The model under review builds one solid part; all positions refer to its coordinate system, in mm. Face numbers are marked on the shaded views. A direction names the side the tool comes from. Coordinates: 2 decimals unless noted, no trailing zeros. Write each loop counter-clockwise with the first axis right and the second up, starting at its lowest first coordinate (ties: lowest second). Pieces come first, ordered by that corner, then holes.
1) For line 1 (X direction, y = -3, z = 0); line 2 (Z direction, x = 0, y = -3.75); line 3 (Y direction, x = 0, z = 0.95), list the stretches that pass through material, from the lowest coordinate up.
2) For P1, Ø6, axis at y = -6.5, z = -4, coming from the +X side; P2, Ø1.5, axis at x = -1, z = 3.5, coming from the +Y side; P3, Ø6, axis at x = 4, z = -4, coming from the -Y side, all flat-tipped, find the tip position at first contact; note any pin that passes through.
3) Add section D-D, the plane x = 0. Give the number of separate pieces and of enclosed holes in the cut face, then the cut area to 4 significant figures.
4) Add section A-A, the plane y = -5.25. State the section outline as (x, z) points, then the cut area to 3 significant figures.
5) Add section C-C, the plane z = 2.25. State the section outline as (x, y) points.
6) Add section B-B, the plane x = 1.5. State the section outline as (y, z) points, then the cut area to 3 significant figures.
7) Machinability: for the marked faces 4, 5, 6 and 7, which of the approach directions +Z, -Z, +X, -X, +Y, -Y give a long, thin tool a straight path to every point of the face, cutting with its end or side? Answer none if there is none.
8) Mouldability with a two-part tool opening along Z and no side actions: class the marked faces 1, 2 and 3 as released by +Z, released by -Z, zero draft, split by the parting line, or undercut.
Autodesk Inventor part; units mm, degrees
ref_plane "YZ Plane" through (0, 0, 0) normal (1, 0, 0) x (0, 1, 0)
ref_plane "XZ Plane" through (0, 0, 0) normal (0, 1, 0) x (-1, 0, 0)
ref_plane "XY Plane" through (0, 0, 0) normal (0, 0, 1) x (1, 0, 0)
sketch "Sketch1" plane through (0, 0, 0) normal (0, 1, 0) x (-1, 0, 0)
  circle A0 centre (0, 0) radius 5.25
  dimension "d0" = 10.5
extrude "Extrusion1" add sketch "Sketch1" against normal blind 12
sketch "Sketch2" plane through (0, 0, 0) normal (0, 1, 0) x (1, 0, 0)
  circle A0 centre (0, 0) radius 4
  dimension "d3" = 8
extrude "Extrusion2" cut sketch "Sketch2" against normal blind 10
sketch "Sketch3" plane through (0, 0, 0) normal (0, 0, 1) x (1, 0, 0)
  point P0 (0, 0)
sketch "Sketch4" plane through (0, 0, 0) normal (0, 0, 1) x (1, 0, 0)
  circle A0 centre (0, 0) radius 0.75
  circle A1 centre (0, 0) radius 1.25
  line L0 (-1.25, 0) -> (-1.25, -10)
  line L1 (-1.25, -10) -> (1.25, -10)
  line L2 (1.25, -10) -> (1.25, 0)
  dimension "d6" = 1.5
  dimension "d7" = 2.5
  dimension "d8" = 10
extrude "Extrusion3" add sketch "Sketch4" along normal mid plane 2 contours L2 L1 L0 A1
sketch "Sketch5" plane through (0, 0, 1) normal (0, 0, 1) x (1, 0, 0)
  circle A0 centre (0, 0) radius 0.75
  circle A1 centre (0, 0) radius 1.25
extrude "Extrusion4" add sketch "Sketch5" along normal mid plane 0.5
extrude "Extrusion5" add sketch "Sketch5" along normal blind 0.5
mirror "Mirror1" about plane through (0, 0, 0) normal (0, 0, 1) of "Extrusion4"
sketch "Sketch6" plane through (0, -12, 0) normal (0, -1, 0) x (1, 0, 0)
  circle A0 centre (0, 0) radius 5.25
extrude "Extrusion6" cut sketch "Sketch6" against normal blind 4
sketch "Sketch7" plane through (0, -8, 0) normal (0, -1, 0) x (1, 0, 0)
  circle A0 centre (0, 0) radius 4
extrude "Extrusion7" add sketch "Sketch7" against normal blind 1
sketch "Sketch8" plane through (0, -8, 0) normal (0, -1, 0) x (1, 0, 0)
  circle A0 centre (0, 0) radius 1.25
  dimension "d19" = 2.5
extrude "Extrusion8" add sketch "Sketch8" along normal blind 2
sketch "Sketch9" plane through (0, 0, 0) normal (0, 0, 1) x (1, 0, 0)
  line L0 (-1.25, -10) -> (1.25, -10)
  line L1 (1.25, -8) -> (-1.25, -8)
  circle A0 centre (0, -9) radius 0.6
  point P0 (0, 0)
  point P1 (0, -8)
  point P2 (0, -10)
  dimension "d23" = 1.2
extrude "Extrusion9" cut sketch "Sketch9" along normal through all both and the other way through all
properties part number "Cylinder_10.5mm"
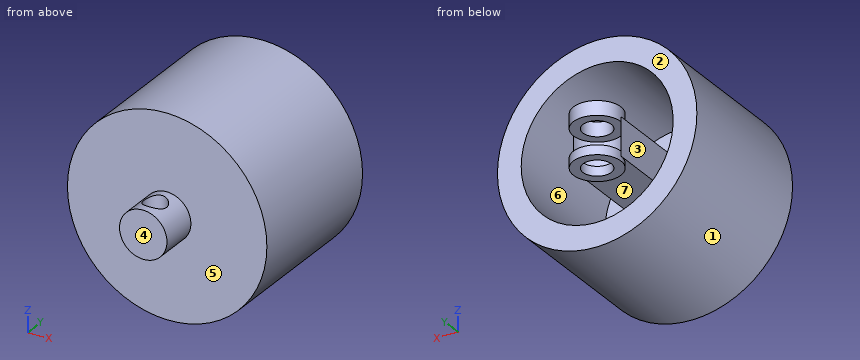
Geometry results:
1. line 1: x = -5.25 to -4, -1.25 to 1.25, 4 to 5.25
1. line 2: z = -5.25 to -4, -1 to 1, 4 to 5.25
1. line 3: y = -10 to -9.6, -8.4 to -0.75, 0.75 to 1.25
2. P1: stops at x = 5.15
2. P2: stops at y = 0
2. P3: stops at y = -8
3. separate pieces: 4
3. enclosed holes: 0
3. area: 42.75 mm2
4. outline: circle Ø10.5 at (0, 0); (-1.25, -1) - (1.25, -1) - (1.25, 1) - (-1.25, 1) - close; hole circle Ø8 at (0, 0)
4. area: 41.3 mm2
5. outline: (-4.74, -8) - (4.74, -8) - (4.74, 0) - (3.31, 0) - (3.31, -7) - (-3.31, -7) - (-3.31, 0) - (-4.74, 0) - close
6. outline: (-8, -5.03) - (0, -5.03) - (0, -3.71) - (-7, -3.71) - (-7, 3.71) - (0, 3.71) - (0, 5.03) - (-8, 5.03) - close
6. area: 28.6 mm2
7. face 4: +Z, -Z, +X, -X, -Y
7. face 5: -Y
7. face 6: +Y
7. face 7: none
8. face 1: split by the parting line
8. face 2: zero draft
8. face 3: undercut
